Part print with two shaded views. Sizes in mm from the minimum x, y, z corner. A direction names the side the tool comes from. Round coordinates to 2 decimals unless told otherwise and drop trailing zeros. Write each loop counter-clockwise with the first axis right and the second up, starting at its lowest first coordinate (ties: lowest second). Pieces come first, ordered by that corner, then holes.
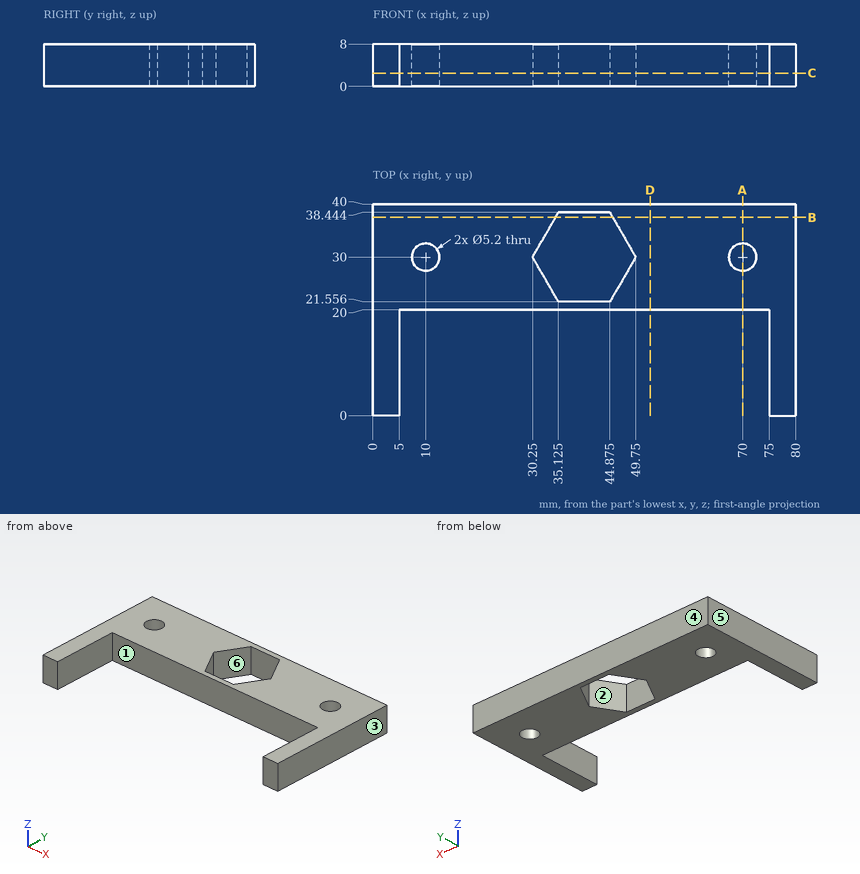
Q1. Which spindle directions (+Z, -Z, +X, -X, +Y, -Y) get a long thin tool onto all of the face, cutting with end or side? Do the marked faces 1, 2 and 3. Say none if no direction does.
Values follow:
face 1: +Z, -Z, -Y
face 2: +Z, -Z
face 3: +Z, -Z, +X, +Y, -Y
Q2. Drop flat-ended pins along their axis: pin 1 (6 mm diameter, centred on x = 10, y = 30, fed in from -Z); pin 2 (4 mm diameter, centred on x = 70, y = 30, fed in from -Z); pin 3 (4 mm diameter, centred on x = 71.5, z = 6.5, fed in from -Y). Give the stop position or say it passes through.
Values follow:
pin 1: stops at z = 0
pin 2: passes through
pin 3: stops at y = 20
Q3. Cut at A-A on x = 70. Write the cut outline in (y, z), plus the area to 3 significant figures.
Values follow:
outline: (20, 0) - (27.4, 0) - (27.4, 8) - (20, 8) - close; (32.6, 0) - (40, 0) - (40, 8) - (32.6, 8) - close
area: 118 mm2
Q4. Mould opens along X. For the marked faces 4, 5 and 6 say: +X half, -X half, draft (parallel to the pull), parting line (faces both ways), or undercut.
Values follow:
face 4: draft
face 5: -X half
face 6: undercut
Q5. Cut at B-B on y = 37.5. Write the cut outline in (x, z).
Values follow:
outline: (0, 0) - (34.58, 0) - (34.58, 8) - (0, 8) - close; (45.42, 0) - (80, 0) - (80, 8) - (45.42, 8) - close
Q6. Cut at D-D on x = 52.5. Write the cut outline in (y, z).
Values follow:
outline: (20, 0) - (40, 0) - (40, 8) - (20, 8) - close
Q7. Wall check: L1, parallel to X at y = 30, z = 2; L2, parallel to X at y = 6, z = 2; L3, parallel to Y at x = 70, z = 5.25. Give the ranges that are in metal, low to high.
Values follow:
L1: x = 0 to 7.4, 12.6 to 30.25, 49.75 to 67.4, 72.6 to 80
L2: x = 0 to 5, 75 to 80
L3: y = 20 to 27.4, 32.6 to 40
Q8. Cut at C-C on z = 2.5. State how many separate pieces and enclosed holes the cut face has, plus the area to 3 significant figures.
Values follow:
separate pieces: 1
enclosed holes: 3
area: 1,510 mm2
